from build123d import *

# Parameters (mm, degrees)
SKETCH2_W           = 12.7
SKETCH2_H           = 23.876
BOSS_EXTRUDE1_DEPTH = 1.524
SKETCH3_W           = 12.7
SKETCH3_H           = 25.4
BOSS_EXTRUDE2_DEPTH = 1.524
FILLET1_R           = 2.54
SKETCH4_R           = 1.651
CUT_EXTRUDE1_DEPTH  = 39.517993004
SKETCH5_R           = 1.651
CUT_EXTRUDE2_DEPTH  = 1.524


with BuildPart() as part:
    # Sketch2 → Boss-Extrude1 (new body)
    with BuildSketch(Plane.XY):
        with Locations((-12.183996683, 11.938)):
            Rectangle(SKETCH2_W, SKETCH2_H)
    extrude(amount=BOSS_EXTRUDE1_DEPTH)

    # Sketch3 → Boss-Extrude2 (add)
    with BuildSketch(Plane.XZ):
        with Locations((-12.183996683, 12.7)):
            Rectangle(SKETCH3_W, SKETCH3_H)
    extrude(amount=BOSS_EXTRUDE2_DEPTH)

    # Fillet1
    fillet1_edges = [part.edges().sort_by_distance(p)[0] for p in [
        (-12.183996683, 0, 1.524),
    ]]
    fillet(fillet1_edges, radius=FILLET1_R)

    # Sketch4 → Cut-Extrude1 (cut, through all)
    with BuildSketch(Plane.XY.offset(1.524)):
        with Locations((-12.183996683, 11.176)):
            Circle(SKETCH4_R)
    extrude(amount=-CUT_EXTRUDE1_DEPTH, mode=Mode.SUBTRACT)

    # Sketch5 → Cut-Extrude2 (cut)
    with BuildSketch(Plane(origin=(0, 0, 0), x_dir=(1, 0, 0), z_dir=(0, 1, 0))):
        with Locations(Location((-12.183996683, -12.7, 0), (0, 0, 180))):
            Circle(SKETCH5_R)
    extrude(amount=-CUT_EXTRUDE2_DEPTH, mode=Mode.SUBTRACT)


solid = part.part
Here's how the part is built. I have some questions about the finished solid (model axes, mm). A direction names the side the tool comes from. Round coordinates to 2 decimals unless told otherwise and drop trailing zeros. Write each loop counter-clockwise with the first axis right and the second up, starting at its lowest first coordinate (ties: lowest second). Pieces come first, ordered by that corner, then holes.
1. Suppose I cut it at A-A (x = -9). List the corners of the cut face in (y, z) for me, and give its area (3 significant figures).
2. Suppose I cut it at C-C (y = 8.5). List the corners of the cut face in (x, z) for me, and give its area (3 significant figures).
3. I need wall thicknesses on L1, parallel to Y at x = -17, z = 17; L2, parallel to Z at x = -11, y = 21; L3, parallel to Z at x = -15, y = 1.75. Which ranges of each line are inside material? Lowest first, please.
4. For faces 5 (the flat face through (-12, 13, 1.524)), 6 (the cylindrical face through (-12.399, 12.813, 0.773)), which set-ups out of +Z, -Z, +X, -X, +Y, -Y let a thin tool reach every point of the face, with its end or its side?
5. If we mould it in two halves opening along Z, with no side actions, what happens to faces 1 (the cylindrical face through (-10.97, -0.75, 13.82)), 2 (the flat face through (-12, 23.876, 1)), 3 (the cylindrical face through (-12.1, 0.76, 2.25)), 4 (the flat face through (-15, 11, 0))? For each: released by +Z, released by -Z, zero draft, split by the parting line, or undercut.
6. Suppose I cut it at B-B (z = 12.7). List the corners of the cut face in (x, y) for me (3 decimals), and give its area (3 significant figures).
7. Will these pins go through, and if not, where does the flat tip stop? pin 1 Ø4 at (x, z) = (-12.18, 12.7) entering from +Y; pin 2 Ø4 at (y, z) = (18.5, 4.5) entering from +X.
Answer sheet:
1. outline: (-1.52, 0) - (23.88, 0) - (23.88, 1.52) - (2.54, 1.52) arc R2.54 cw to (0, 4.06) - (0, 25.4) - (-1.52, 25.4) - close
1. area: 76.5 mm2
2. outline: (-18.53, 0) - (-5.83, 0) - (-5.83, 1.52) - (-18.53, 1.52) - close
2. area: 19.4 mm2
3. L1: y = -1.52 to 0
3. L2: z = 0 to 1.52
3. L3: z = 0 to 1.65
4. face 5: +Z, +X, -X, +Y
4. face 6: +Z, -Z
5. face 1: undercut
5. face 2: zero draft
5. face 3: released by +Z
5. face 4: released by -Z
6. outline: (-18.534, -1.524) - (-13.835, -1.524) - (-13.835, 0) - (-18.534, 0) - close; (-10.533, -1.524) - (-5.834, -1.524) - (-5.834, 0) - (-10.533, 0) - close
6. area: 14.3 mm2
7. pin 1: stops at y = 0
7. pin 2: passes through
